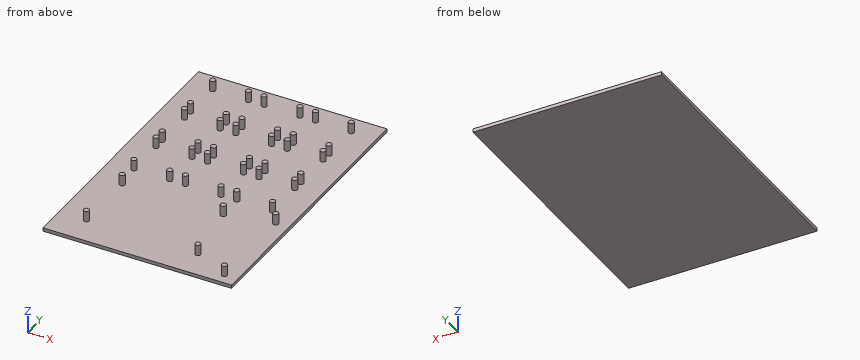
from build123d import *

# Parameters (mm, degrees)
SKETCH1_W           = 139.7
SKETCH1_H           = 209.55
BOSS_EXTRUDE1_DEPTH = 2.54
SKETCH2_R           = 2
BOSS_EXTRUDE2_DEPTH = 7.9375
SKETCH3_R           = 2
BOSS_EXTRUDE3_DEPTH = 7.9375


with BuildPart() as part:
    # Sketch1 → Boss-Extrude1 (new body)
    with BuildSketch(Plane.XY):
        Rectangle(SKETCH1_W, SKETCH1_H)
    extrude(amount=BOSS_EXTRUDE1_DEPTH)

    # Sketch2 → Boss-Extrude2 (add)
    with BuildSketch(Plane.XY.offset(2.54)):
        with Locations((-51.349999916, 14.125)):
            Circle(SKETCH2_R)
        with Locations((-24.849999916, 14.125)):
            Circle(SKETCH2_R)
        with Locations((-24.849999916, -15.875)):
            Circle(SKETCH2_R)
        with Locations((-51.349999916, -15.875)):
            Circle(SKETCH2_R)
        with Locations((13.250000084, 14.125)):
            Circle(SKETCH2_R)
        with Locations((-13.249999916, 14.125)):
            Circle(SKETCH2_R)
        with Locations((-13.249999916, -15.875)):
            Circle(SKETCH2_R)
        with Locations((13.250000084, -15.875)):
            Circle(SKETCH2_R)
        with Locations((51.350000084, 14.125)):
            Circle(SKETCH2_R)
        with Locations((24.850000084, 14.125)):
            Circle(SKETCH2_R)
        with Locations((24.850000084, -15.875)):
            Circle(SKETCH2_R)
        with Locations((51.350000084, -15.875)):
            Circle(SKETCH2_R)
        with Locations((13.250000084, 52.225)):
            Circle(SKETCH2_R)
        with Locations((-13.249999916, 52.225)):
            Circle(SKETCH2_R)
        with Locations((-13.249999916, 22.225)):
            Circle(SKETCH2_R)
        with Locations((13.250000084, 22.225)):
            Circle(SKETCH2_R)
        with Locations((51.350000084, 52.225)):
            Circle(SKETCH2_R)
        with Locations((24.850000084, 52.225)):
            Circle(SKETCH2_R)
        with Locations((24.850000084, 22.225)):
            Circle(SKETCH2_R)
        with Locations((51.350000084, 22.225)):
            Circle(SKETCH2_R)
        with Locations((13.250000084, 90.325)):
            Circle(SKETCH2_R)
        with Locations((-13.249999916, 90.325)):
            Circle(SKETCH2_R)
        with Locations((-13.249999916, 60.325)):
            Circle(SKETCH2_R)
        with Locations((13.250000084, 60.325)):
            Circle(SKETCH2_R)
        with Locations((51.350000084, 90.325)):
            Circle(SKETCH2_R)
        with Locations((24.850000084, 90.325)):
            Circle(SKETCH2_R)
        with Locations((24.850000084, 60.325)):
            Circle(SKETCH2_R)
        with Locations((51.350000084, 60.325)):
            Circle(SKETCH2_R)
        with Locations((-24.849999916, 52.225)):
            Circle(SKETCH2_R)
        with Locations((-51.349999916, 52.225)):
            Circle(SKETCH2_R)
        with Locations((-51.349999916, 22.225)):
            Circle(SKETCH2_R)
        with Locations((-24.849999916, 22.225)):
            Circle(SKETCH2_R)
        with Locations((-24.849999916, 90.325)):
            Circle(SKETCH2_R)
        with Locations((-51.349999916, 90.325)):
            Circle(SKETCH2_R)
        with Locations((-51.349999916, 60.325)):
            Circle(SKETCH2_R)
        with Locations((-24.849999916, 60.325)):
            Circle(SKETCH2_R)
    extrude(amount=BOSS_EXTRUDE2_DEPTH)

    # Sketch3 → Boss-Extrude3 (add)
    with BuildSketch(Plane.XY.offset(2.54)):
        with Locations((-49.5, -83.225)):
            Circle(SKETCH3_R)
        with Locations((33.02, -83.225)):
            Circle(SKETCH3_R)
        with Locations((60, -96.5125)):
            Circle(SKETCH3_R)
        with Locations((60, -27.3125)):
            Circle(SKETCH3_R)
        with Locations((25.4, -35.025)):
            Circle(SKETCH3_R)
        with Locations((-49.5, -35.025)):
            Circle(SKETCH3_R)
    extrude(amount=BOSS_EXTRUDE3_DEPTH)


solid = part.part
Verification items for the finished model (mm, model axes). Coordinates: 2 decimals unless noted, no trailing zeros. Loops run counter-clockwise (first coordinate to the right, second up) from the corner with the lowest first, then second, coordinate; pieces in that order, holes last. Notation, with made-up numbers: M -33,74.5 L -28,74.5 A26 cw -28,107.5 Z; hole C 19.25,1 d9. An arc over 180 degrees is marked long. One line per item, written item: value.
1. Section check C-C on z = 7.25. Give the number of separate pieces and of enclosed holes in the cut face, plus the area to 3 significant figures.
Answers follow:
separate pieces: 42
enclosed holes: 0
area: 528 mm^2
2. Gauge pin test, flat end, axial feed: P1, Ø6, axis at x = -45.5, z = 9, coming from the -Y side. Record the tip position at first contact, or that the pin passes through.
Answers follow:
P1: y = -84.96
3. Section check A-A on x = 5. Record the cut outline in (y, z) (3 decimals).
Answers follow:
outline: M -104.775,0 L 104.775,0 L 104.775,2.54 L -104.775,2.54 Z
4. Material ranges on line 1 along X through (y, z) = (14, 3.25); line 2 along Y through (x, z) = (51, 3.75); line 3 along Y through (x, z) = (51.5, 5.25), recorded low to high. Write a range as from..to.
Answers follow:
line 1: -53.35..-49.35, -26.85..-22.85, -15.25..-11.25, 11.25..15.25, 22.85..26.85, 49.35..53.35
line 2: -17.84..-13.91, 12.16..16.09, 20.26..24.19, 50.26..54.19, 58.36..62.29, 88.36..92.29
line 3: -17.87..-13.88, 12.13..16.12, 20.23..24.22, 50.23..54.22, 58.33..62.32, 88.33..92.32
5. Section check B-B on y = 8.5. Record the cut outline in (x, z), plus the area to 3 significant figures.
Answers follow:
outline: M -69.85,0 L 69.85,0 L 69.85,2.54 L -69.85,2.54 Z
area: 355 mm^2
